Study the drawing (mm; zero at the part's minimum x, y, z) and answer. A direction names the side the tool comes from. Give positions to 0.01 mm unless a question says otherwise; leave off trailing zeros. Order: outer loops, then holes, each group sorted by start corner. A loop starts at its lowest first (then second) coordinate and runs counter-clockwise, first axis right, second up.
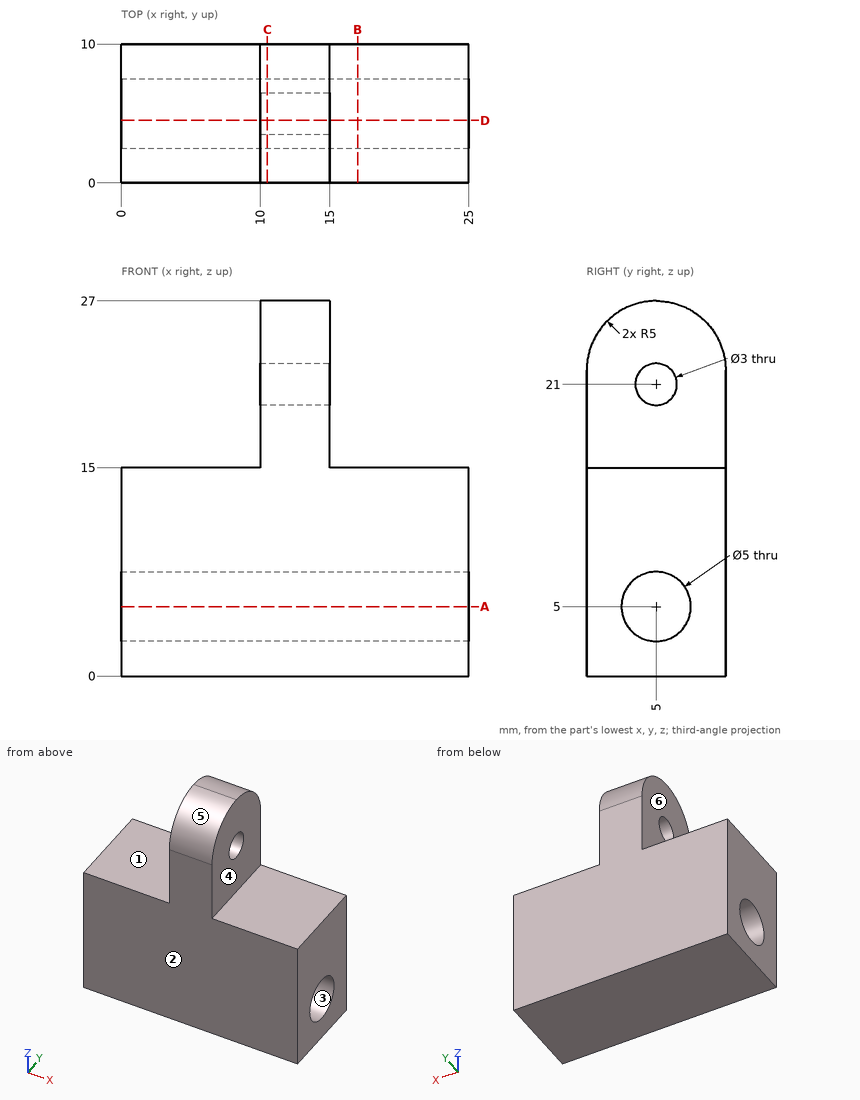
1) Find section A-A (z = 5). Write down the section's boundary in (x, y), then the cut area to 3 significant figures.
Geometry says:
outline: (0, 0) - (25, 0) - (25, 2.5) - (0, 2.5) - close; (0, 7.5) - (25, 7.5) - (25, 10) - (0, 10) - close
area: 125 mm2
2) Given P1, Ø5, axis at y = 7.5, z = 19, coming from the -X side; P2, Ø2, axis at x = 15.5, y = 7, coming from the -Z side; P3, Ø3, axis at x = 6, y = 7.5, coming from the +Z side; P4, Ø2.5, axis at y = 5, z = 21, coming from the +X side, each flat-ended and moving along its own axis, determine where each tip first touches the part or whether it passes through.
Geometry says:
P1: stops at x = 10
P2: stops at z = 0
P3: stops at z = 15
P4: passes through
3) A tool of negligible diameter and unlimited length cuts with its end or side. For the marked faces 4, 5 and 6, from which of +Z, -Z, +X, -X, +Y, -Y can it reach the whole face along a straight path? Write none if from no direction.
Geometry says:
face 4: +Z, +X, +Y, -Y
face 5: +Z, +X, -X, -Y
face 6: +Z, -X, +Y, -Y
4) Find section C-C (x = 10.5). Count the separate pieces of the cut face and the enclosed holes in it, then the cut area to 3 significant figures.
Geometry says:
separate pieces: 1
enclosed holes: 2
area: 233 mm2
5) Find section B-B (x = 17). Write down the section's boundary in (y, z).
Geometry says:
outline: (0, 0) - (10, 0) - (10, 15) - (0, 15) - close; hole circle Ø5 at (5, 5)
6) Find section D-D (y = 4.5). Write down the section's boundary in (x, z) (1 decimal), then the cut area to 3 significant figures.
Geometry says:
outline: (0, 0) - (25, 0) - (25, 2.6) - (0, 2.6) - close; (0, 7.4) - (25, 7.4) - (25, 15) - (15, 15) - (15, 19.6) - (10, 19.6) - (10, 15) - (0, 15) - close; (10, 22.4) - (15, 22.4) - (15, 27) - (10, 27) - close
area: 298 mm2
7) Straight lines are drawn through the part: probe 1 along Z at (x, y) = (22.25, 3); probe 2 along Y at (x, z) = (11.35, 21); probe 3 along Y at (x, z) = (16.25, 5). For each, find the intervals that lie inside material, in ascending order.
Geometry says:
probe 1: z = 0 to 3.5, 6.5 to 15
probe 2: y = 0 to 3.5, 6.5 to 10
probe 3: y = 0 to 2.5, 7.5 to 10
8) For a pull along Z with two mould halves and no side action, classify the marked faces 1, 2 and 3 as +Z half, -Z half, draft (parallel to the pull), parting line (faces both ways), or undercut.
Geometry says:
face 1: +Z half
face 2: draft
face 3: undercut
